```python
from build123d import *

# Parameters (mm, degrees)
BOX024_W          = 5
BOX024_H          = 12.5
BOX024_DEPTH      = 5
CYLINDER002_R     = 2.5
CYLINDER002_DEPTH = 5
BOX005_W          = 5
BOX005_H          = 22
BOX005_DEPTH      = 1.9
BOX004_W          = 5
BOX004_H          = 22
BOX004_DEPTH      = 1.9
BOX001_W          = 57.7
BOX001_H          = 57.7
BOX001_DEPTH      = 0.5


with BuildPart() as cube:
    # Box024 → Box024 (new body)
    with BuildSketch(Plane(origin=(27.35, 0, 0), x_dir=(1, 0, 0), z_dir=(0, 0, 1))):
        with Locations((2.5, 6.25)):
            Rectangle(BOX024_W, BOX024_H)
    extrude(amount=BOX024_DEPTH)


with BuildPart() as cylinder001:
    # Cylinder002 → Cylinder002 (new body)
    with BuildSketch(Plane(origin=(29.85, 12.5, 0), x_dir=(1, 0, 0), z_dir=(0, 0, 1))):
        Circle(CYLINDER002_R)
    extrude(amount=CYLINDER002_DEPTH)


with BuildPart() as box005:
    # Box005 → Box005 (new body)
    with BuildSketch(Plane(origin=(54.7, 18.85, 1.9), x_dir=(1, 0, 0), z_dir=(0, 0, 1))):
        with Locations((2.5, 11)):
            Rectangle(BOX005_W, BOX005_H)
    extrude(amount=BOX005_DEPTH)


with BuildPart() as box004:
    # Box004 → Box004 (new body)
    with BuildSketch(Plane(origin=(0, 18.85, 1.9), x_dir=(1, 0, 0), z_dir=(0, 0, 1))):
        with Locations((2.5, 11)):
            Rectangle(BOX004_W, BOX004_H)
    extrude(amount=BOX004_DEPTH)


with BuildPart() as cut008:
    # Box001 → Box001 (new body)
    with BuildSketch(Plane(origin=(1, 1, 1.9), x_dir=(1, 0, 0), z_dir=(0, 0, 1))):
        with Locations((28.85, 28.85)):
            Rectangle(BOX001_W, BOX001_H)
    extrude(amount=BOX001_DEPTH)

    # Cut003: cut Box004
    add(box004.part, mode=Mode.SUBTRACT)

    # Cut004: cut Box005
    add(box005.part, mode=Mode.SUBTRACT)

    # Cut007: cut Cylinder001
    add(cylinder001.part, mode=Mode.SUBTRACT)

    # Cut008: cut Cube
    add(cube.part, mode=Mode.SUBTRACT)


solid = cut008.part
```
Verification items for the finished model (mm, model axes). Round coordinates to 2 decimals unless told otherwise and drop trailing zeros. Order: outer loops, then holes, each group sorted by start corner. A loop starts at its lowest first (then second) coordinate and runs counter-clockwise, first axis right, second up.
1) Cross-section at D-D, the plane y = 24. Record the cut outline in (x, z), plus the area to 4 significant figures.
Geometry says:
outline: (5, 1.9) - (54.7, 1.9) - (54.7, 2.4) - (5, 2.4) - close
area: 24.85 mm2
2) Material ranges on line 1 (X direction, y = 34, z = 2.1); line 2 (Y direction, x = 28.5, z = 2); line 3 (Y direction, x = 28, z = 2.2), recorded low to high.
Geometry says:
line 1: x = 5 to 54.7
line 2: y = 14.6 to 58.7
line 3: y = 14.18 to 58.7
3) Cross-section at C-C, the plane x = 29.85. Record the cut outline in (y, z), plus the area to 4 significant figures.
Geometry says:
outline: (15, 1.9) - (58.7, 1.9) - (58.7, 2.4) - (15, 2.4) - close
area: 21.85 mm2
4) Draft check along X on faces 1 (the cylindrical face through (29.9, 15, 2.1)), 2 (the flat face through (29, 30, 2.4)). Enter one of: +X half, -X half, draft (parallel to the pull), parting line (faces both ways), or undercut.
Geometry says:
face 1: undercut
face 2: draft
5) Cross-section at A-A, the plane y = 11.5. Record the cut outline in (x, z), plus the area to 4 significant figures.
Geometry says:
outline: (1, 1.9) - (27.35, 1.9) - (27.35, 2.4) - (1, 2.4) - close; (32.35, 1.9) - (58.7, 1.9) - (58.7, 2.4) - (32.35, 2.4) - close
area: 26.35 mm2
6) Cross-section at B-B, the plane z = 2.05. Record the cut outline in (x, y), plus the area to 3 significant figures.
Geometry says:
outline: (1, 1) - (27.35, 1) - (27.35, 12.5) arc R2.5 cw to (32.35, 12.5) - (32.35, 1) - (58.7, 1) - (58.7, 18.85) - (54.7, 18.85) - (54.7, 40.85) - (58.7, 40.85) - (58.7, 58.7) - (1, 58.7) - (1, 40.85) - (5, 40.85) - (5, 18.85) - (1, 18.85) - close
area: 3,090 mm2
